```python
from build123d import *

# Parameters (mm, degrees)
SKETCH2_R           = 38.5
SKETCH2_R_2         = 32.5
BOSS_EXTRUDE1_DEPTH = 5


with BuildPart() as part:
    # Sketch1 → Revolve1 (revolve)
    with BuildSketch(Plane.XY, mode=Mode.PRIVATE) as revolve1_sk:
        Polygon((2, 0), (2, 50), (32.5, 108), (38.5, 108), (8, 50), (8, 0), align=None)
    revolve(revolve1_sk.sketch.rotate(Axis((0, 0, 0), (0, 1, 0)), 90), axis=Axis((0, 0, 0), (0, 1, 0)))

    # Sketch2 → Boss-Extrude1 (add)
    with BuildSketch(Plane(origin=(0, 108, 0), x_dir=(1, 0, 0), z_dir=(0, 1, 0))):
        with Locations(Location((0, 0, 0), (0, 0, 270))):
            Circle(SKETCH2_R)
        Circle(SKETCH2_R_2, mode=Mode.SUBTRACT)
    extrude(amount=-BOSS_EXTRUDE1_DEPTH)


solid = part.part
```
Source: CAD feature listing. Evaluate the final solid. Frame: model axes, mm. A direction names the side the tool comes from. Round coordinates to 2 decimals unless told otherwise and drop trailing zeros. Order: outer loops, then holes, each group sorted by start corner. A loop starts at its lowest first (then second) coordinate and runs counter-clockwise, first axis right, second up. Notation, with made-up numbers: (40.5, 89.25) -> (95.5, 89.25) arc R12 cw to (95.5, 96.25) -> close; hole circle Ø10 at (12.25, -16). An arc over 180 degrees is marked (long way). One line per item, written item: value. Start each with the question number.
Q1. Material intervals for probe 1 along X at (y, z) = (21, 0); probe 2 along Z at (x, y) = (-19, 93); probe 3 along Z at (x, y) = (6.5, 87), sorted ascending.
Q2. Section query B-B (z = 0). Return the cut outline in (x, y), plus the area to 3 significant figures.
Q3. Pin query (flat end, axial travel): pin 1 (10 mm diameter, centred on y = 81.5, z = -6, fed in from +X); pin 2 (8 mm diameter, centred on x = 18.5, y = 87, fed in from +Z); pin 3 (3 mm diameter, centred on y = 24.5, z = -6.5, fed in from -X) (3 decimals). Return the tip coordinate at first contact, or that it passes through.
Q4. Access query for faces 1 (the flat face through (17, 103, -32)), 2 (the flat face through (20, 108, -26)). Directions: +Z, -Z, +X, -X, +Y, -Y. A direction counts if a zero-diameter tool reaches every point of the face in a straight line with its end or side. Return the directions, or none.
Q5. Section query D-D (y = 65). Return the cut outline in (x, z), plus the area to 3 significant figures.
Q6. Section query A-A (x = 0). Return the cut outline in (y, z).
Q7. Section query C-C (y = 90.5). Return the cut outline in (x, z).
Q8. Draft query along Z for faces 3 (the conical face through (-4.228, 72.962, -13.425)), 4 (the flat face through (2, 0, -2)), 5 (the cylindrical face through (-37.584, 105.535, -8.346)), 6 (the cylindrical face through (2, 25, 0)). Return one class per face: pulls with the +Z half, pulls with the -Z half, needs draft (parallel to the pull), parting line crosses it, or undercut.
Findings below:
1. probe 1: -8 to -2, 2 to 8
1. probe 2: -24 to -15.64, 15.64 to 24
1. probe 3: -26.68 to -20.45, 20.45 to 26.68
2. outline: (-38.5, 103) -> (-35.87, 103) -> (-8, 50) -> (-8, 0) -> (-2, 0) -> (-2, 50) -> (-32.5, 108) -> (-38.5, 108) -> close; (2, 0) -> (8, 0) -> (8, 50) -> (35.87, 103) -> (38.5, 103) -> (38.5, 108) -> (32.5, 108) -> (2, 50) -> close
2. area: 1,310 mm²
3. pin 1: x = 26.7
3. pin 2: z = 24.33
3. pin 3: x = -6.245
4. face 1: -Y
4. face 2: +Z, -Z, +X, -X, +Y
5. outline: circle Ø31.78 at (0, 0); hole circle Ø19.78 at (0, 0)
5. area: 486 mm²
6. outline: (0, -8) -> (50, -8) -> (103, -35.87) -> (103, -38.5) -> (108, -38.5) -> (108, -32.5) -> (50, -2) -> (0, -2) -> close; (0, 2) -> (50, 2) -> (108, 32.5) -> (108, 38.5) -> (103, 38.5) -> (103, 35.87) -> (50, 8) -> (0, 8) -> close
7. outline: circle Ø58.59 at (0, 0); hole circle Ø46.59 at (0, 0)
8. face 3: undercut
8. face 4: needs draft
8. face 5: parting line crosses it
8. face 6: undercut
